Part model, mm, in its own coordinate system. Give positions to 0.01 mm unless a question says otherwise; leave off trailing zeros. Order: outer loops, then holes, each group sorted by start corner. A loop starts at its lowest first (then second) coordinate and runs counter-clockwise, first axis right, second up.
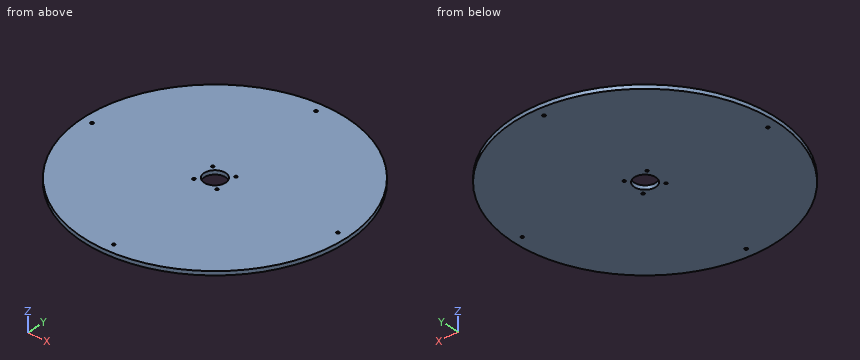
from build123d import *

# Parameters (mm, degrees)
SKETCH089_R           = 398.87
PAD013_DEPTH          = 12
SKETCH090_R           = 4.25
POCKET056_DEPTH       = 0.001
POCKET056_DEPTH_BACK  = 12.001
SKETCH091_R           = 32.5
POCKET057_DEPTH       = 0.001
POCKET057_DEPTH_BACK  = 12.001
SKETCH092_R           = 4.5
POCKET058_DEPTH       = 2256.478091
POCKET058_DEPTH_BACK  = 2268.478091
POLARPATTERN016_COUNT = 4


with BuildPart() as part:
    # Sketch089 → Pad013 (new body)
    with BuildSketch(Plane.XY):
        Circle(SKETCH089_R)
    extrude(amount=PAD013_DEPTH)

    # Sketch090 → Pocket056 (cut, two sides)
    with BuildSketch(Plane.XY) as pocket056_sk:
        with Locations((34.56, 34.56)):
            Circle(SKETCH090_R)
        with Locations((-34.56, 34.56)):
            Circle(SKETCH090_R)
        with Locations((-34.56, -34.56)):
            Circle(SKETCH090_R)
        with Locations((34.56, -34.56)):
            Circle(SKETCH090_R)
    extrude(amount=-POCKET056_DEPTH, mode=Mode.SUBTRACT)
    extrude(pocket056_sk.sketch, amount=POCKET056_DEPTH_BACK, mode=Mode.SUBTRACT)

    # Sketch091 → Pocket057 (cut, two sides)
    with BuildSketch(Plane.XY) as pocket057_sk:
        Circle(SKETCH091_R)
    extrude(amount=-POCKET057_DEPTH, mode=Mode.SUBTRACT)
    extrude(pocket057_sk.sketch, amount=POCKET057_DEPTH_BACK, mode=Mode.SUBTRACT)

    # Sketch092 → Pocket058 (cut, two sides)
    with BuildSketch(Plane(origin=(368.87, 0, 0), x_dir=(1, 0, 0), z_dir=(0, 0, 1))) as pocket058_sk:
        Circle(SKETCH092_R)
    pocket058 = extrude(amount=-POCKET058_DEPTH, mode=Mode.SUBTRACT) + extrude(pocket058_sk.sketch, amount=POCKET058_DEPTH_BACK, mode=Mode.SUBTRACT)

    # PolarPattern016: Pocket058 ×4 about axis
    polarpattern016_axis = Axis((0, 0, 0), (0, 0, 1))
    for i in range(1, POLARPATTERN016_COUNT):
        add(pocket058.rotate(polarpattern016_axis, i * 360 / POLARPATTERN016_COUNT), mode=Mode.SUBTRACT)


solid = part.part
Item 1: Band-saw the part on A-A on z = 3. Give the number of separate pieces and of enclosed holes in the cut face, plus the area to 3 significant figures.
Item 2: Band-saw the part on C-C on y = 305. List the corners of the cut face in (x, z), plus the area to 3 significant figures.
Item 3: Drop flat-ended pins along their axis: P1, Ø7.5, axis at x = 34.56, y = -34.56, coming from the -Z side; P2, Ø3, axis at x = 183, z = 8.5, coming from the -Y side; P3, Ø4, axis at y = 209, z = 3.5, coming from the -X side; P4, Ø5, axis at y = 315, z = 6.5, coming from the -X side. Give the stop position or say it passes through.
Item 4: Drill centre lines: probe 1 along Y at (x, z) = (34.56, 4.75); probe 2 along X at (y, z) = (368.87, 8). Where is each one in solid material? Low to high.
Item 5: Band-saw the part on B-B on y = 156. List the corners of the cut face in (x, z).
Working result:
1. separate pieces: 1
1. enclosed holes: 9
1. area: 496,000 mm2
2. outline: (-257.05, 0) - (257.05, 0) - (257.05, 12) - (-257.05, 12) - close
2. area: 6,170 mm2
3. P1: passes through
3. P2: stops at y = -355.18
3. P3: stops at x = -340.95
3. P4: stops at x = -247.87
4. probe 1: y = -397.37 to -38.81, -30.31 to 30.31, 38.81 to 397.37
4. probe 2: x = -151.76 to -4.5, 4.5 to 151.76
5. outline: (-367.1, 0) - (367.1, 0) - (367.1, 12) - (-367.1, 12) - close
